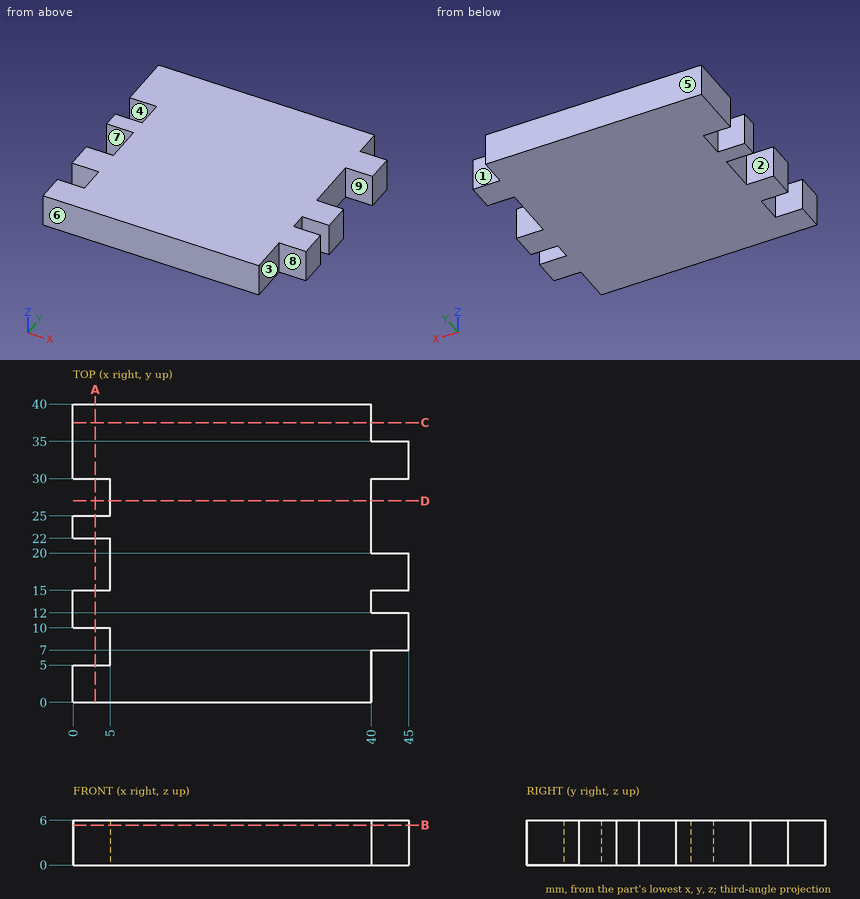
For this review, use the dimensioned drawing (mm, ordinates from the lowest corner) and the shaded views. A direction names the side the tool comes from. Coordinates: 2 decimals unless noted, no trailing zeros. Order: outer loops, then holes, each group sorted by start corner. A loop starts at its lowest first (then second) coordinate and runs counter-clockwise, first axis right, second up. Notation, with made-up numbers: (39.25, -20) -> (52.25, -20) arc R22 cw to (52.25, -10) -> close; hole circle Ø7 at (59.5, -24). An arc over 180 degrees is marked (long way). One line per item, written item: value. Start each with the question number.
Q1. Take a section at B-B, the plane z = 5.35. State the section outline as (x, y) points, then the cut area to 3 significant figures.
Q2. For probe 1 along Y at (x, z) = (41, 4.9); probe 2 along X at (y, z) = (19.5, 2.8); probe 3 along X at (y, z) = (23, 5.65), list the stretches that pass through material, from the lowest coordinate up.
Q3. Take a section at D-D, the plane y = 27. State the section outline as (x, z) points, then the cut area to 3 significant figures.
Q4. Insertion check: pin 1 Ø2.5 at (x, z) = (42, 3.5) entering from +Y; pin 2 Ø1.5 at (y, z) = (28, 1.5) entering from -X; pin 3 Ø1.5 at (y, z) = (13, 3.5) entering from +X. Each pin has a flat end and moves straight along its axis. Give the tip position at first contact, or say it passes through.
Q5. Take a section at A-A, the plane x = 3. State the section outline as (y, z) points, then the cut area to 3 significant figures.
Q6. Tool access review of the marked faces 5, 6, 7, 8 and 9: name each direction out of +Z, -Z, +X, -X, +Y, -Y from which nothing blocks a thin tool from reaching the whole face with its end or side.
Q7. Mouldability with a two-part tool opening along Y and no side actions: class the marked faces 1, 2, 3 and 4 as pulls with the +Y half, pulls with the -Y half, needs draft (parallel to the pull), parting line crosses it, or undercut.
Q8. Take a section at C-C, the plane y = 37.5. State the section outline as (x, z) points, then the cut area to 3 significant figures.
Values follow:
1. outline: (0, 0) -> (40, 0) -> (40, 7) -> (45, 7) -> (45, 12) -> (40, 12) -> (40, 15) -> (45, 15) -> (45, 20) -> (40, 20) -> (40, 30) -> (45, 30) -> (45, 35) -> (40, 35) -> (40, 40) -> (0, 40) -> (0, 30) -> (5, 30) -> (5, 25) -> (0, 25) -> (0, 22) -> (5, 22) -> (5, 15) -> (0, 15) -> (0, 10) -> (5, 10) -> (5, 5) -> (0, 5) -> close
1. area: 1,590 mm2
2. probe 1: y = 7 to 12, 15 to 20, 30 to 35
2. probe 2: x = 5 to 45
2. probe 3: x = 0 to 40
3. outline: (5, 0) -> (40, 0) -> (40, 6) -> (5, 6) -> close
3. area: 210 mm2
4. pin 1: stops at y = 35
4. pin 2: stops at x = 5
4. pin 3: stops at x = 40
5. outline: (0, 0) -> (5, 0) -> (5, 6) -> (0, 6) -> close; (10, 0) -> (15, 0) -> (15, 6) -> (10, 6) -> close; (22, 0) -> (25, 0) -> (25, 6) -> (22, 6) -> close; (30, 0) -> (40, 0) -> (40, 6) -> (30, 6) -> close
5. area: 138 mm2
6. face 5: +Z, -Z, +X, -X, +Y
6. face 6: +Z, -Z, +X, -X, -Y
6. face 7: +Z, -Z, -X
6. face 8: +Z, -Z, +X, -Y
6. face 9: +Z, -Z, +X
7. face 1: pulls with the +Y half
7. face 2: undercut
7. face 3: needs draft
7. face 4: undercut
8. outline: (0, 0) -> (40, 0) -> (40, 6) -> (0, 6) -> close
8. area: 240 mm2
